Input: part model. Units: mm. Frame: model coordinates. Face numbers are marked on the shaded views. Coordinates: 2 decimals unless noted, no trailing zeros. Loops run counter-clockwise (first coordinate to the right, second up) from the corner with the lowest first, then second, coordinate; pieces in that order, holes last. Notation, with made-up numbers: (-5, 26) - (21, 26) arc R10 cw to (21, 31) - close; hole circle Ø6 at (-5, -33.75). An arc over 180 degrees is marked (long way). Use one line per item in the form item = value.
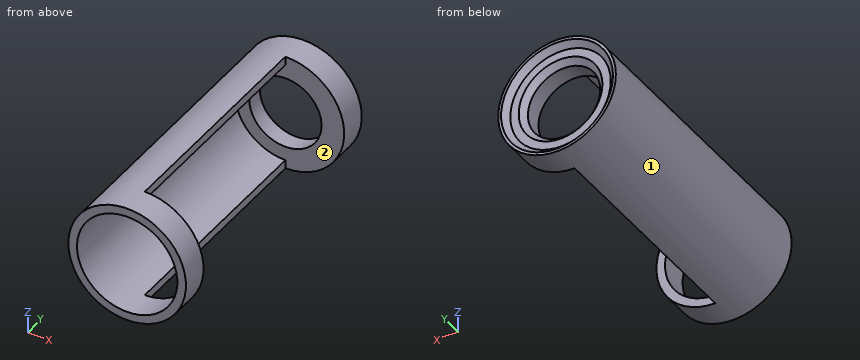
Autodesk Inventor part; units mm, degrees
ref_plane "YZ Plane" through (0, 0, 0) normal (1, 0, 0) x (0, 1, 0)
ref_plane "XZ Plane" through (0, 0, 0) normal (0, 1, 0) x (-1, 0, 0)
ref_plane "XY Plane" through (0, 0, 0) normal (0, 0, 1) x (1, 0, 0)
sketch "Sketch1" plane through (0, 0, 0) normal (0, 1, 0) x (-1, 0, 0)
  circle A0 centre (0, 0) radius 13.0175
  circle A1 centre (0, 0) radius 11.1125
  line L0 (0, 13.0175) -> (0, 11.1125)
  line L1 (0, -11.1125) -> (0, -13.0175)
  circle A2 centre (0, 0) radius 8
  dimension "d0" = 26.035
  dimension "d1" = 22.225
  dimension "d6" = 16
extrude "Extrusion1" add sketch "Sketch1" along normal blind 6.35 contours A0 L1 A1 L0 | L0 A1 L1 A0
extrude "Extrusion2" add sketch "Sketch1" against normal blind 25.4 contours A0 L1 A1 L0 picked at (12.2737, -0.9656)
mirror "Mirror1" about plane through (-6.5087, -25.4, 0) normal (0, -1, 0) of "Extrusion2", "Extrusion1"
extrude "Extrusion3" add sketch "Sketch1" along normal blind 5.08 contours A1
chamfer "Chamfer1" distance 1.27 angle 45 2 edges at (11.1125, 6.35, 0) (8, 5.08, 0)
properties part number "Electronics HousingV2_3DPrint"
Q1. Ray query, line 1 along Y through (x, z) = (9.5, -1.75); line 2 along X through (y, z) = (-42, 0); line 3 along Z through (x, y) = (-4, -9.5). Return the intervals inside material, ascending. Write a range as [from, to].
Check values:
line_1 = [0, 5.08]
line_2 = [-13.02, -11.11]
line_3 = [-12.39, -10.37], [10.37, 12.39]
Q2. Cut plane A-A, the plane z = 0. Give the number of separate pieces and of enclosed holes in the cut face, then the cut area to 3 significant figures.
Check values:
separate_pieces = 3
enclosed_holes = 0
area = 174 mm²
Q3. First-contact query: P1, Ø12, axis at y = -16.5, z = 9.5, coming from the -X side; P2, Ø1.5, axis at y = -30.5, z = 11.5, coming from the +X side; P3, Ø6.5, axis at x = 5.5, z = -0.5, coming from the +Y side; P4, Ø14.5, axis at x = 0, z = 0, coming from the -Y side. Flat tips, straight axial feed; report the tip coordinate or a pass-through.
Check values:
P1 = -12.54
P2 = 0
P3 = 4.58
P4 = through
Q4. Cut plane B-B, the plane y = -33. Return loops of the section in (x, z) (1 decimal), then the cut area to 3 significant figures.
Check values:
outline = (0, -13) - (0, -11.1) arc R11.1 cw to (0, 11.1) - (0, 13) arc R13 ccw to start
area = 72.2 mm²
Q5. Pull-direction query (Z, two-part tool) for the marked faces 1 and 2; classes: pulls with the +Z half, pulls with the -Z half, needs draft (parallel to the pull), parting line crosses it, or undercut.
Check values:
face_1 = parting line crosses it
face_2 = undercut
